Input: part model. Units: mm. Frame: model coordinates. Face numbers are marked on the shaded views. Coordinates: 2 decimals unless noted, no trailing zeros. Order: outer loops, then holes, each group sorted by start corner. A loop starts at its lowest first (then second) coordinate and runs counter-clockwise, first axis right, second up. Notation, with made-up numbers: (-10, 65) -> (23, 65) arc R19 cw to (23, 96) -> close; hole circle Ø4 at (42.5, 7.25). An arc over 180 degrees is marked (long way). Answer as CSV lines item,"result".
from build123d import *

# Parameters (mm, degrees)
SCHIZZO1_R                   = 5
ESTRUSIONE_ESTRUSIONE1_DEPTH = 115
ESTRUSIONE_ESTRUSIONE2_DEPTH = 6
TAGLIO_ESTRUSIONE1_REACH     = 118.245
SCHIZZO3_R                   = 6
SMUSSO1_SIZE                 = 1


with BuildPart() as part:
    # Schizzo1 → Estrusione-Estrusione1 (new body)
    with BuildSketch(Plane(origin=(0, 0, 0), x_dir=(0, 0, -1), z_dir=(1, 0, 0))):
        Circle(SCHIZZO1_R)
    extrude(amount=ESTRUSIONE_ESTRUSIONE1_DEPTH)

    # Schizzo2 → Estrusione-Estrusione2 (add, symmetric)
    with BuildSketch(Plane(origin=(0, 0, 0), x_dir=(1, 0, 0), z_dir=(0, 1, 0))):
        with BuildLine():
            Line((0, 12), (12, 12))
            ThreePointArc((12, 12), (24, 0), (12, -12))
            Line((12, -12), (0, -12))
            ThreePointArc((0, -12), (-12, 0), (0, 12))
        make_face()
    extrude(amount=ESTRUSIONE_ESTRUSIONE2_DEPTH, both=True)

    # Schizzo3 → Taglio-Estrusione1 (cut, up to next)
    with BuildSketch(Plane(origin=(0, 6, 0), x_dir=(1, 0, 0), z_dir=(0, 1, 0)), mode=Mode.PRIVATE) as taglio_estrusione1_sk1:
        with Locations(Location((0, 0, 0), (0, 0, 270))):
            Circle(SCHIZZO3_R)
    taglio_estrusione1_tool1 = extrude(taglio_estrusione1_sk1.sketch, amount=-TAGLIO_ESTRUSIONE1_REACH, mode=Mode.PRIVATE) & part.part
    add(taglio_estrusione1_tool1.solids().sort_by_distance((0, 6, 0))[0], mode=Mode.SUBTRACT)

    # Smusso1
    smusso1_edges = [part.edges().sort_by_distance(p)[0] for p in [
        (0, 6, -6),
        (0, -6, -6),
        (115, 0, 5),
    ]]
    chamfer(smusso1_edges, length=SMUSSO1_SIZE)


solid = part.part
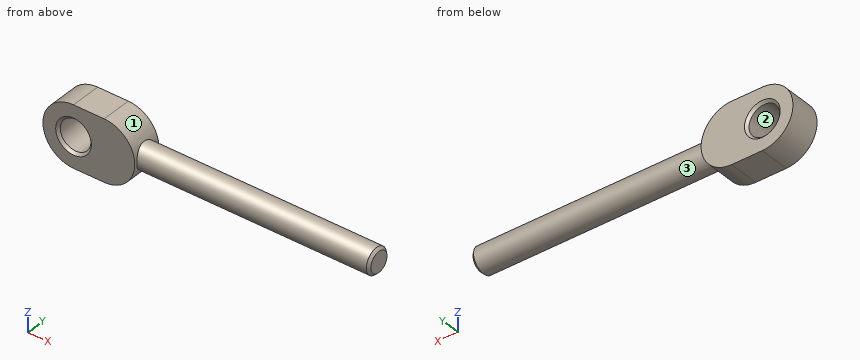
1. Cut plane B-B (y = 0). Return the cut outline in (x, z), plus the area to 3 significant figures.
Findings:
outline,"(0, -12) -> (12, -12) arc R12 ccw to (22.91, -5) -> (114, -5) -> (115, -4) -> (115, 4) -> (114, 5) -> (22.91, 5) arc R12 ccw to (12, 12) -> (0, 12) arc R12 ccw to start; hole circle Ø12 at (0, 0)"
area,"1,540 mm2"
2. Cut plane C-C (z = -8.75). Return the cut outline in (x, y).
Findings:
outline,"(-8.21, -6) -> (20.21, -6) -> (20.21, 6) -> (-8.21, 6) -> close"
3. Mould query, pull axis X, two halves, no side actions, for the marked faces 1, 2 and 3. Classes: released by +X, released by -X, zero draft, split by the parting line, or undercut.
Findings:
face 1,"released by +X"
face 2,"undercut"
face 3,"zero draft"
4. Ray query, line 1 along X through (y, z) = (0.75, 0); line 2 along X through (y, z) = (-5.5, -2); line 3 along Y through (x, z) = (59.5, -0.5). Return the intervals inside material, ascending.
Findings:
line 1,"x = -12 to -6, 6 to 115"
line 2,"x = -11.83 to -6.18, 6.18 to 23.83"
line 3,"y = -4.97 to 4.97"
5. Cut plane A-A (z = 0). Return the cut outline in (x, y).
Findings:
outline,"(-12, -6) -> (-7, -6) -> (-6, -5) -> (-6, 5) -> (-7, 6) -> (-12, 6) -> close; (6, -5) -> (7, -6) -> (24, -6) -> (24, -5) -> (114, -5) -> (115, -4) -> (115, 4) -> (114, 5) -> (24, 5) -> (24, 6) -> (7, 6) -> (6, 5) -> close"
6. Contact query for flat-ended pins moving along their axis: pin 1 (1.5 mm diameter, centred on x = 80.5, z = -6.5, fed in from +Y); pin 2 (5 mm diameter, centred on y = 0.5, z = 8, fed in from -X); pin 3 (1.5 mm diameter, centred on x = 42.5, y = 0.5, fed in from -Z). Output: stop coordinate, or through.
Findings:
pin 1,"passes through"
pin 2,"stops at x = -10.67"
pin 3,"stops at z = -5"
